Geometry check sheet. Reference: the model listing, model coordinates, mm. Face numbers are marked on the shaded views. A direction names the side the tool comes from. Give positions to 0.01 mm unless a question says otherwise; leave off trailing zeros. Loops run counter-clockwise (first coordinate to the right, second up) from the corner with the lowest first, then second, coordinate; pieces in that order, holes last.
1. Cross-section at A-A, the plane y = 0. Record the cut outline in (x, z), plus the area to 3 significant figures.
2. Release check for a two-part mould opening along Y. For the marked faces 1, 2, 3 and 4 record: +Y half, -Y half, draft (parallel to the pull), parting line (faces both ways), or undercut.
3. Tool access check on the marked faces 5, 6, 7 and 8. Record the directions out of +Z, -Z, +X, -X, +Y, -Y that give a thin tool (end or side, any length) a straight path to the whole face; none if there is none.
4. Cross-section at B-B, the plane x = -16. Record the cut outline in (y, z).
5. Cross-section at C-C, the plane z = -15.75. Record the cut outline in (x, y).
6. Material ranges on L1, parallel to Y at x = -16, z = 2.2; L2, parallel to Y at x = 11, z = -15.5; L3, parallel to X at y = 13.1, z = -10, recorded low to high.
7. Cross-section at D-D, the plane x = -81. Record the cut outline in (y, z), plus the area to 3 significant figures.
8. Go/stop test with flat-tipped pins: pin 1 Ø4.5 at (x, y) = (12, 49) entering from -Z; pin 2 Ø4 at (x, y) = (-9, 44.5) entering from -Z; pin 3 Ø1 at (y, z) = (31, -2.5) entering from +X; pin 4 Ø8 at (y, z) = (31.5, -10) entering from +X. Record where each tip stops, or that it passes through.
from build123d import *

# Parameters (mm, degrees)
F0_R      = 2.5
F1_DEPTH  = 3
F2_W      = 45
F2_H      = 3
F3_DEPTH  = 22
F5_DEPTH  = 3
F7_DEPTH  = 22
F8_R      = 1.6
F9_DEPTH  = 6
F10_R     = 3
F11_DEPTH = 25
F12_DEPTH = 30


with BuildPart() as f1:
    # F0 (on Top) → F1 (new body)
    with BuildSketch(Plane.XY):
        Polygon((18, -10), (109, -10), (109, 10), (22.5, 53.6), (-22.5, 53.6), (-109, 10), (-109, -10), (3, -10), align=None)
        with Locations((-99, 0)):
            Circle(F0_R, mode=Mode.SUBTRACT)
        with Locations((99, 0)):
            Circle(F0_R, mode=Mode.SUBTRACT)
    extrude(amount=F1_DEPTH)

    # F2 (on face) → F3 (join)
    with BuildSketch(Plane(origin=(0, 0, 0), x_dir=(1, 0, 0), z_dir=(0, 0, -1))):
        with Locations((0, -52.1)):
            Rectangle(F2_W, F2_H)
    extrude(amount=F3_DEPTH)

    # F4 (on face) → F5 (join)
    with BuildSketch(Plane(origin=(0, 0, 0), x_dir=(1, 0, 0), z_dir=(0, 0, -1))):
        Polygon((89, -13), (-89, -13), (-89, -10), (-109, -10), (-103.048165, -13), (-53.449541, -38), (53.449541, -38), (103.048165, -13), (109, -10), (89, -10), align=None)
    extrude(amount=F5_DEPTH)

    # F6 (on face) → F7 (join)
    with BuildSketch(Plane(origin=(0, 0, -3), x_dir=(1, 0, 0), z_dir=(0, 0, -1))):
        Polygon((89, -13), (-89, -13), (-89, -10), (-109, -10), (-97.09633, -16), (97.09633, -16), (109, -10), (89, -10), align=None)
    extrude(amount=F7_DEPTH)

    # F8 (on face) → F9 (cut)
    with BuildSketch(Plane.XZ.offset(-10)):
        with Locations((-99, -10)):
            Circle(F8_R)
        with Locations((99, -10)):
            Circle(F8_R)
    extrude(amount=-F9_DEPTH, mode=Mode.SUBTRACT)

    # F10 (on face) → F11 (cut)
    with BuildSketch(Plane.XY.offset(3)):
        with Locations((-16, 45.6)):
            Circle(F10_R)
        with Locations((-16, 22.6)):
            Circle(F10_R)
        with Locations((16, 22.6)):
            Circle(F10_R)
        with Locations((16, 45.6)):
            Circle(F10_R)
    extrude(amount=-F11_DEPTH, mode=Mode.SUBTRACT)

    # F10 (on face) → F12 (cut)
    with BuildSketch(Plane.XY.offset(3)):
        with Locations((-16, 45.6)):
            Circle(F10_R)
        with Locations((-16, 22.6)):
            Circle(F10_R)
        with Locations((16, 22.6)):
            Circle(F10_R)
        with Locations((16, 45.6)):
            Circle(F10_R)
    extrude(amount=-F12_DEPTH, mode=Mode.SUBTRACT)


solid = f1.part
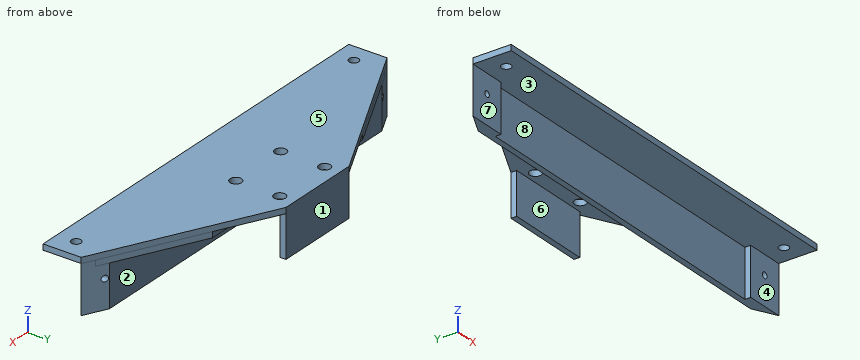
Result:
1. outline: (-109, 0) - (-101.5, 0) - (-101.5, 3) - (-109, 3) - close; (-96.5, 0) - (96.5, 0) - (96.5, 3) - (-96.5, 3) - close; (101.5, 0) - (109, 0) - (109, 3) - (101.5, 3) - close
1. area: 624 mm2
2. face 1: +Y half
2. face 2: undercut
2. face 3: draft
2. face 4: -Y half
3. face 5: +Z, +X, -X, +Y, -Y
3. face 6: -Z, +X, -X
3. face 7: -Z, +X, -X, -Y
3. face 8: -Z, -Y
4. outline: (-10, 0) - (13, 0) - (13, -25) - (16, -25) - (16, -3) - (19.6, -3) - (19.6, 3) - (-10, 3) - close; (25.6, -3) - (38, -3) - (38, 0) - (42.6, 0) - (42.6, 3) - (25.6, 3) - close; (48.6, 0) - (50.6, 0) - (50.6, -22) - (53.6, -22) - (53.6, 3) - (48.6, 3) - close
5. outline: (-109, 10) - (-89, 10) - (-89, 13) - (89, 13) - (89, 10) - (109, 10) - (97.1, 16) - (-97.1, 16) - close; (-22.5, 50.6) - (22.5, 50.6) - (22.5, 53.6) - (-22.5, 53.6) - close
6. L1: y = -10 to 19.6, 25.6 to 42.6, 48.6 to 53.6
6. L2: y = 13 to 16, 50.6 to 53.6
6. L3: x = -102.85 to -100.6, -97.4 to 97.4, 100.6 to 102.85
7. outline: (-10, 0) - (13, 0) - (13, -25) - (16, -25) - (16, -3) - (24.11, -3) - (24.11, 3) - (-10, 3) - close
7. area: 202 mm2
8. pin 1: stops at z = -22
8. pin 2: stops at z = 0
8. pin 3: stops at x = 68.33
8. pin 4: passes through
